```python
from build123d import *
from OCP.BRepFilletAPI import BRepFilletAPI_MakeChamfer
from build123d.topology import SkipClean

# Parameters (mm, degrees)
BOSS_EXTRU_1_DEPTH           = 15
ENL_V_START                  = -1.3
ESQUISSE2_R                  = 9.6
ENL_V_MAT_EXTRU_1_DEPTH      = 29.4
ENL_V_MAT_EXTRU_2_DEPTH      = 36.895542898805694
ENL_V_MAT_EXTRU_2_DEPTH_BACK = 36.895542898805694
BOSS_EXTRU_2_DEPTH           = 3
ESQUISSE6_R                  = 1.7
ENL_V_MAT_EXTRU_3_DEPTH      = 30.000000000000014
CHANFREIN1_SIZE              = 5
CHANFREIN1_SIZE2             = 7
CHANFREIN2_SIZE              = 7
CHANFREIN2_SIZE2             = 6
CHANFREIN3_START             = 12.698865856
CHANFREIN3_OUTLINE_W         = 11
CHANFREIN3_OUTLINE_H         = 12.000000000000002
CHANFREIN3_DEPTH             = 4.301134144
CHANFREIN4_START             = 12.698865856
CHANFREIN4_OUTLINE_W         = 11
CHANFREIN4_OUTLINE_H         = 12.000000000000002
CHANFREIN4_DEPTH             = 4.301134144
CHANFREIN5_START             = -17
CHANFREIN5_OUTLINE_W         = 11
CHANFREIN5_OUTLINE_H         = 12.000000000000002
CHANFREIN5_DEPTH             = 4.301134144
CHANFREIN6_START             = -17
CHANFREIN6_OUTLINE_W         = 11
CHANFREIN6_OUTLINE_H         = 12.000000000000002
CHANFREIN6_DEPTH             = 4.301134144
ENL_V_START_2                = -13.5
ENL_V_MAT_EXTRU_4_DEPTH      = 4


with BuildPart() as part:
    # Esquisse1 → Boss.-Extru.1 (new body)
    with BuildSketch(Plane.XY):
        Polygon((-16.000000000000007, 11.000000000000002), (15.999999999999993, 11.000000000000002), (15.999999999999996, -11), (-16, -11), align=None)
    extrude(amount=BOSS_EXTRU_1_DEPTH)

    # Esquisse2 → Enlèv. mat.-Extru.1 (cut)
    with BuildSketch(Plane(origin=(15.999999999999996, 2.52e-15, 0), x_dir=(0, 0, -1), z_dir=(1, 1.6e-16, 0)).offset(ENL_V_START)):
        with Locations((-15, -1.73e-15)):
            Circle(ESQUISSE2_R)
    extrude(amount=-ENL_V_MAT_EXTRU_1_DEPTH, mode=Mode.SUBTRACT)

    # Esquisse4 → Enlèv. mat.-Extru.2 (cut, two sides: drawn at the far end of the back side and taken through both)
    with SkipClean():  # the faces are left unmerged after this step: merging them gives an invalid solid
        with BuildSketch(Plane(origin=(-14.700000000000001, -2.32e-15, 0), x_dir=(0, 0, -1), z_dir=(1, 1.6e-16, 0)).offset(-ENL_V_MAT_EXTRU_2_DEPTH_BACK)):
            with BuildLine():
                Line((-7.3999999999999995, -5.865151319446073), (-7.3999999999999995, 5.865151319446073))
                ThreePointArc((-7.3999999999999995, 5.865151319446073), (-10.76593886833709, 8.615841591704243), (-15.000000000000032, 9.599999999999998))
                Line((-15.000000000000032, 9.599999999999998), (-15, -9.600000000000001))
                ThreePointArc((-15, -9.600000000000001), (-10.765938868337066, -8.615841591704251), (-7.3999999999999995, -5.865151319446073))
            make_face()
        extrude(amount=ENL_V_MAT_EXTRU_2_DEPTH + ENL_V_MAT_EXTRU_2_DEPTH_BACK, mode=Mode.SUBTRACT)

    # Esquisse5 → Boss.-Extru.2 (add)
    with BuildSketch(Plane(origin=(0, 0, 0), x_dir=(-1, 0, 0), z_dir=(0, 0, -1))):
        Polygon((7.000000000000008, -11), (-6.999999999999992, -11.000000000000002), (-6.999999999999991, -20.999999999999993), (7.000000000000009, -20.999999999999996), align=None)
        Polygon((7.000000000000006, 11.000000000000002), (-6.999999999999994, 11), (-6.999999999999992, 20.999999999999996), (7.000000000000008, 20.999999999999996), align=None)
    extrude(amount=-BOSS_EXTRU_2_DEPTH)

    # Esquisse6 → Enlèv. mat.-Extru.3 (cut, through all)
    with BuildSketch(Plane.XY.offset(3)):
        with Locations((0, -15.999999999999996)):
            Circle(ESQUISSE6_R)
        with Locations((8.7e-16, 15.999999999999996)):
            Circle(ESQUISSE6_R)
    extrude(amount=-ENL_V_MAT_EXTRU_3_DEPTH, mode=Mode.SUBTRACT)

    # Chanfrein1: one chamfer whose edges measure the first distance from different faces: ONE call of the kernel's chamfer builder (chamfer() names one face for all edges)
    chanfrein1_edges_1 = [part.edges().sort_by_distance(p)[0] for p in [
        (6.999999999999991, -20.999999999999993, 1.5),
    ]]
    chanfrein1_side_1 = [part.faces().sort_by_distance(p)[0] for p in [
        (-9.13e-15, -20.999999999999993, 1.5),
    ]]
    chanfrein1_edges_2 = [part.edges().sort_by_distance(p)[0] for p in [
        (-7.000000000000008, 20.999999999999996, 1.5),
    ]]
    chanfrein1_side_2 = [part.faces().sort_by_distance(p)[0] for p in [
        (-8.24e-15, 20.999999999999996, 1.5),
    ]]
    chanfrein1 = BRepFilletAPI_MakeChamfer(part.part.solid().wrapped)
    for e in chanfrein1_edges_1:
        chanfrein1.Add(CHANFREIN1_SIZE, CHANFREIN1_SIZE2, e.wrapped, chanfrein1_side_1[0].wrapped)  # the first distance lies on this face
    for e in chanfrein1_edges_2:
        chanfrein1.Add(CHANFREIN1_SIZE, CHANFREIN1_SIZE2, e.wrapped, chanfrein1_side_2[0].wrapped)  # the first distance lies on this face
    add(Compound.cast(chanfrein1.Shape()), mode=Mode.REPLACE)

    # Chanfrein2: one chamfer whose edges measure the first distance from different faces: ONE call of the kernel's chamfer builder (chamfer() names one face for all edges)
    chanfrein2_edges_1 = [part.edges().sort_by_distance(p)[0] for p in [
        (6.999999999999992, 20.999999999999996, 1.5),
    ]]
    chanfrein2_side_1 = [part.faces().sort_by_distance(p)[0] for p in [
        (6.999999999999993, 15.999999999999998, 1.5),
    ]]
    chanfrein2_edges_2 = [part.edges().sort_by_distance(p)[0] for p in [
        (-7.000000000000009, -20.999999999999996, 1.5),
    ]]
    chanfrein2_side_2 = [part.faces().sort_by_distance(p)[0] for p in [
        (-7.000000000000009, -15.999999999999998, 1.5),
    ]]
    chanfrein2 = BRepFilletAPI_MakeChamfer(part.part.solid().wrapped)
    for e in chanfrein2_edges_1:
        chanfrein2.Add(CHANFREIN2_SIZE, CHANFREIN2_SIZE2, e.wrapped, chanfrein2_side_1[0].wrapped)  # the first distance lies on this face
    for e in chanfrein2_edges_2:
        chanfrein2.Add(CHANFREIN2_SIZE, CHANFREIN2_SIZE2, e.wrapped, chanfrein2_side_2[0].wrapped)  # the first distance lies on this face
    add(Compound.cast(chanfrein2.Shape()), mode=Mode.REPLACE)

    # Chanfrein3: read off the stored shape, not the designer's step
    # Chanfrein3 outline → Chanfrein3 (cut)
    with BuildSketch(Plane(origin=(0, 0, 0), x_dir=(0.7964473354898962, 0.4591284639882932, 0.39353868341853704), z_dir=(0.6047078979069521, -0.6047078979069521, -0.5183210553488161)).offset(CHANFREIN3_START)):
        with Locations((6.5, 8)):
            Rectangle(CHANFREIN3_OUTLINE_W, CHANFREIN3_OUTLINE_H)
    extrude(amount=CHANFREIN3_DEPTH, mode=Mode.SUBTRACT)

    # Chanfrein4: read off the stored shape, not the designer's step
    # Chanfrein4 outline → Chanfrein4 (cut)
    with BuildSketch(Plane(origin=(0, 0, 0), x_dir=(0.7964473354898962, -0.45912846398829327, 0.39353868341853704), z_dir=(0.6047078979069521, 0.6047078979069522, -0.5183210553488161)).offset(CHANFREIN4_START)):
        with Locations((6.5, -8)):
            Rectangle(CHANFREIN4_OUTLINE_W, CHANFREIN4_OUTLINE_H)
    extrude(amount=CHANFREIN4_DEPTH, mode=Mode.SUBTRACT)

    # Chanfrein5: read off the stored shape, not the designer's step
    # Chanfrein5 outline → Chanfrein5 (cut)
    with BuildSketch(Plane(origin=(0, 0, 0), x_dir=(0.7964473354898962, 0.45912846398829327, -0.39353868341853704), z_dir=(0.6047078979069521, -0.6047078979069522, 0.5183210553488161)).offset(CHANFREIN5_START)):
        with Locations((-6.5, 8)):
            Rectangle(CHANFREIN5_OUTLINE_W, CHANFREIN5_OUTLINE_H)
    extrude(amount=CHANFREIN5_DEPTH, mode=Mode.SUBTRACT)

    # Chanfrein6: read off the stored shape, not the designer's step
    # Chanfrein6 outline → Chanfrein6 (cut)
    with BuildSketch(Plane(origin=(0, 0, 0), x_dir=(0.7964473354898959, -0.4591284639882932, -0.3935386834185371), z_dir=(0.6047078979069522, 0.6047078979069521, 0.5183210553488161)).offset(CHANFREIN6_START)):
        with Locations((-6.5, -8)):
            Rectangle(CHANFREIN6_OUTLINE_W, CHANFREIN6_OUTLINE_H)
    extrude(amount=CHANFREIN6_DEPTH, mode=Mode.SUBTRACT)

    # Esquisse7 → Enlèv. mat.-Extru.4 (cut)
    with BuildSketch(Plane(origin=(15.999999999999996, 2.52e-15, 0), x_dir=(0, 0, -1), z_dir=(1, 1.6e-16, 0)).offset(ENL_V_START_2)):
        Polygon((-3, -7.571428571428581), (-3, 7.571428571428564), (-7.000000000000009, 11), (-3.000000000000009, 11), (-4.5e-16, 8.428571428571422), (1.83e-15, -8.428571428571436), (-2.999999999999989, -11.000000000000002), (-6.9999999999999885, -11.000000000000002), align=None)
    extrude(amount=-ENL_V_MAT_EXTRU_4_DEPTH, mode=Mode.SUBTRACT)


solid = part.part
```
The listing builds one solid part. Answer for the finished solid, in the listing's coordinates (mm). A direction names the side the tool comes from. Round coordinates to 2 decimals unless told otherwise and drop trailing zeros. Loops run counter-clockwise (first coordinate to the right, second up) from the corner with the lowest first, then second, coordinate; pieces in that order, holes last.
Q1. Which of the six approach directions +Z, -Z, +X, -X, +Y, -Y give full straight-line access (tool end or side, diameter ignored) to faces 1 (the face through (1, 0, 3)), 2 (the face through (-15, 0, 7.4)), 3 (the face through (-7, 13, 1)), 4 (the face through (0, 14, 3))?
Q2. Section A-A, the plane x = 0 is taken. Determine the outline of the cut face in (y, z), then the cut area to 3 significant figures.
Q3. Given pin 1 Ø0.9 at (y, z) = (-12.5, 1.5) entering from +X; pin 2 Ø8 at (x, y) = (-1.5, -4.5) entering from +Z; pin 3 Ø3 at (x, y) = (0.5, 18.5) entering from +Z; pin 4 Ø4 at (x, y) = (-10, 14.5) entering from +Z, each flat-ended and moving along its own axis, determine where each tip first touches the part or whether it passes through.
Q4. Section B-B, the plane y = 16 is taken. Determine the outline of the cut face in (x, z).
Q5. Section D-D, the plane x = 9 is taken. Determine the outline of the cut face in (y, z), then the cut area to 3 significant figures.
Q6. Find the intervals of material crossed by line 1 (Y direction, x = 0, z = 0.7); line 2 (Y direction, x = 0, z = 1.2); line 3 (Z direction, x = -2.5, y = 19), in increasing order.
Q7. For a pull along Z with two mould halves and no side action, classify faces 5 (the face through (-1.5, 0, 2)), 6 (the face through (2.5, 0, 2)), 7 (the face through (-3, 0, 0)), 8 (the face through (7, 12, 1)) as released by +Z, released by -Z, zero draft, split by the parting line, or undercut.
Q8. Section C-C, the plane z = 8.5 is taken. Determine the outline of the cut face in (x, y), then the cut area to 3 significant figures.
Completed:
1. face 1: -Z
1. face 2: +Z, +X, -X
1. face 3: +Z, -Z, -X, +Y
1. face 4: +Z, +X, -X, +Y
2. outline: (-21, 0) - (-17.7, 0) - (-17.7, 3) - (-21, 3) - close; (-14.3, 0) - (-8.43, 0) - (-11, 3) - (-14.3, 3) - close; (-11, 7) - (-7.57, 3) - (7.57, 3) - (11, 7) - (11, 15) - (9.6, 15) arc R9.6 cw to (-9.6, 15) - (-11, 15) - close; (8.43, 0) - (14.3, 0) - (14.3, 3) - (11, 3) - close; (17.7, 0) - (21, 0) - (21, 3) - (17.7, 3) - close
2. area: 153 mm2
3. pin 1: stops at x = 7
3. pin 2: stops at z = 10.54
3. pin 3: stops at z = 3
3. pin 4: passes through
4. outline: (-5.57, 0) - (-1.7, 0) - (-1.7, 3) - (-5.57, 3) - close; (1.7, 0) - (5.29, 0) - (5.29, 3) - (1.7, 3) - close
5. outline: (-11, 0) - (11, 0) - (11, 15) - (9.6, 15) arc R9.6 cw to (-9.6, 15) - (-11, 15) - close
5. area: 185 mm2
6. line 1: y = -21 to -17.7, -14.3 to -9.03, 9.03 to 14.3, 17.7 to 21
6. line 2: y = -21 to -17.7, -14.3 to -9.46, 9.46 to 14.3, 17.7 to 21
6. line 3: z = 0 to 3
7. face 5: undercut
7. face 6: undercut
7. face 7: released by -Z
7. face 8: zero draft
8. outline: (-16, -11) - (16, -11) - (16, -7.06) - (-16, -7.06) - close; (-16, 7.06) - (16, 7.06) - (16, 11) - (-16, 11) - close
8. area: 252 mm2
